Input: part model. Units: mm. Frame: model coordinates. Face numbers are marked on the shaded views. A direction names the side the tool comes from. Give positions to 0.01 mm unless a question says otherwise; leave off trailing zeros. Write each loop counter-clockwise with the first axis right and the second up, starting at its lowest first coordinate (ties: lowest second). Pieces come first, ordered by that corner, then holes.
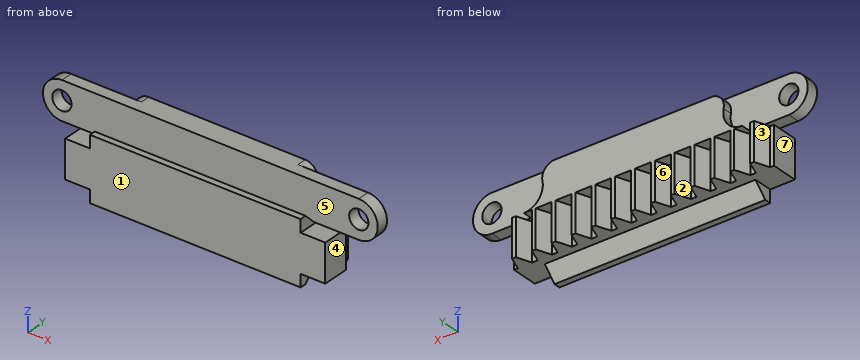
```python
from build123d import *

# Parameters (mm, degrees)
BOSS_EXTRUDE1_DEPTH              = 6
SKETCH4_W                        = 33.355842528
SKETCH4_H                        = 6
BOSS_EXTRUDE3_DEPTH              = 3
BOSS_EXTRUDE4_DEPTH              = 33.355842528
SKETCH17_W                       = 28.5
SKETCH17_H                       = 1.9
BOSS_EXTRUDE11_DEPTH             = 6
SKETCH18_R                       = 1.525
BOSS_EXTRUDE12_DEPTH             = 1.9
SKETCH20_W                       = 34.55751915
SKETCH20_H                       = 1.75
BOSS_EXTRUDE13_DEPTH             = 6
SKETCH21_R                       = 3
CUT_EXTRUDE3_DEPTH               = 1.75
FILLET2_START                    = -9.24613882
FILLET2_DEPTH                    = 1.75
BOSS_EXTRUDE14_REACH             = 49.223
SKETCH22_W                       = 6
SKETCH22_H                       = 3
BOSS_EXTRUDE14_DIRECTION_2_REACH = 49.223
SPLIT1_START                     = -66.92498259
SPLIT1_DEPTH                     = 33.355842528
SPLIT1_START_2                   = -11.14613882
SPLIT1_2_DEPTH                   = 3.65
SPLIT1_3_OUTLINE_R               = 1.525
SPLIT1_3_DEPTH                   = 1.9
SPLIT1_START_3                   = 6.755649514
SPLIT1_4_DEPTH                   = 6
SKETCH26_W                       = 6
SKETCH26_H                       = 2.5
CUT_EXTRUDE4_DEPTH               = 51.815209001
SKETCH27_W                       = 6
SKETCH27_H                       = 0.25
CUT_EXTRUDE5_DEPTH               = 80.093428855


with BuildPart() as part:
    # Sketch1 → Boss-Extrude1 (new body)
    with BuildSketch(Plane(origin=(0, 0, 0.755649514), x_dir=(-1, 0, 0), z_dir=(0, 0, -1))):
        Polygon((31.089725273, -5.24613882), (30.270792245, -7.49613882), (29.667061326, -7.49613882), (29.667061326, -11.24613882), (70.667061326, -11.24613882), (70.827061326, -11.24613882), (70.827061326, -7.49613882), (70.667061326, -7.49613882), (70.222625956, -7.49613882), (69.403692929, -5.24613882), (68.788837073, -5.24613882), (67.969904045, -7.49613882), (67.081033306, -7.49613882), (66.262100279, -5.24613882), (65.647244423, -5.24613882), (64.828311395, -7.49613882), (63.939440656, -7.49613882), (63.120507629, -5.24613882), (62.505651773, -5.24613882), (61.686718745, -7.49613882), (60.797848006, -7.49613882), (59.978914979, -5.24613882), (59.364059123, -5.24613882), (58.545126095, -7.49613882), (57.656255356, -7.49613882), (56.837322329, -5.24613882), (56.222466473, -5.24613882), (55.403533445, -7.49613882), (54.514662706, -7.49613882), (53.695729679, -5.24613882), (53.080873823, -5.24613882), (52.261940795, -7.49613882), (51.373070056, -7.49613882), (50.554137029, -5.24613882), (49.939281173, -5.24613882), (49.120348145, -7.49613882), (48.231477406, -7.49613882), (47.412544379, -5.24613882), (46.797688523, -5.24613882), (45.978755495, -7.49613882), (45.089884756, -7.49613882), (44.270951729, -5.24613882), (43.656095873, -5.24613882), (42.837162845, -7.49613882), (41.948292106, -7.49613882), (41.129359079, -5.24613882), (40.514503223, -5.24613882), (39.695570195, -7.49613882), (38.806699456, -7.49613882), (37.987766429, -5.24613882), (37.372910573, -5.24613882), (36.553977545, -7.49613882), (35.665106806, -7.49613882), (34.846173779, -5.24613882), (34.231317923, -5.24613882), (33.412384895, -7.49613882), (32.523514156, -7.49613882), (31.704581129, -5.24613882), align=None)
    extrude(amount=-BOSS_EXTRUDE1_DEPTH)

    # Sketch4 → Boss-Extrude3 (add)
    with BuildSketch(Plane.XZ.offset(11.24613882)):
        with Locations((-50.247061326, 3.755649514)):
            Rectangle(SKETCH4_W, SKETCH4_H)
    extrude(amount=BOSS_EXTRUDE3_DEPTH)

    # Sketch5 → Boss-Extrude4 (add)
    with BuildSketch(Plane.ZY.offset(66.92498259)):
        Polygon((0.755649514, -11.24613882), (-1.244350486, -13.24613882), (-1.244350486, -14.24613882), (0.755649514, -14.24613882), align=None)
        Polygon((8.755649514, -13.24613882), (8.755649514, -14.24613882), (6.755649514, -14.24613882), (6.755649514, -11.24613882), align=None)
    extrude(amount=-BOSS_EXTRUDE4_DEPTH)

    # Sketch17 → Boss-Extrude11 (add)
    with BuildSketch(Plane.XY.offset(6.755649514)):
        with Locations((-50.247061326, -10.19613882)):
            Rectangle(SKETCH17_W, SKETCH17_H)
    extrude(amount=BOSS_EXTRUDE11_DEPTH)

    # Sketch18 → Boss-Extrude12 (add)
    with BuildSketch(Plane(origin=(0, -9.24613882, 0), x_dir=(1, 0, 0), z_dir=(0, 1, 0))):
        with BuildLine():
            Line((-73.747061326, -6.755649514), (-26.747061326, -6.755649514))
            ThreePointArc((-26.747061326, -6.755649514), (-23.747061326, -9.755649514), (-26.747061326, -12.755649514))
            Line((-26.747061326, -12.755649514), (-73.747061326, -12.755649514))
            ThreePointArc((-73.747061326, -12.755649514), (-76.747061326, -9.755649514), (-73.747061326, -6.755649514))
        make_face()
        with Locations(Location((-73.747061326, -9.755649514, 0), (0, 0, 270))):
            Circle(SKETCH18_R, mode=Mode.SUBTRACT)
        with Locations(Location((-26.747061326, -9.755649514, 0), (0, 0, 270))):
            Circle(SKETCH18_R, mode=Mode.SUBTRACT)
    extrude(amount=-BOSS_EXTRUDE12_DEPTH)

    # Sketch20 → Boss-Extrude13 (add)
    with BuildSketch(Plane.XY.offset(6.755649514)):
        with Locations((-50.246709101, -8.37113882)):
            Rectangle(SKETCH20_W, SKETCH20_H)
    extrude(amount=BOSS_EXTRUDE13_DEPTH)

    # Sketch21 → Cut-Extrude3 (cut)
    with BuildSketch(Plane(origin=(0, -7.49613882, 0), x_dir=(1, 0, 0), z_dir=(0, 1, 0))):
        with Locations((-67.525468676, -9.755649514)):
            Circle(SKETCH21_R)
        with Locations((-32.967949526, -9.755649514)):
            Circle(SKETCH21_R)
    extrude(amount=-CUT_EXTRUDE3_DEPTH, mode=Mode.SUBTRACT)

    # Fillet2: read off the stored shape, not the designer's step
    # Fillet2 outline → Fillet2 (cut)
    with BuildSketch(Plane(origin=(0, 0, 0), x_dir=(1, 0, 0), z_dir=(0, 1, 0)).offset(FILLET2_START)):
        with BuildLine():
            ThreePointArc((-35.907337217, -10.355649514), (-36.317735672, -12.020560578), (-37.866929011, -12.755649514))
            Line((-37.866929011, -12.755649514), (-32.967949526, -12.755649514))
            ThreePointArc((-32.967949526, -12.755649514), (-34.865316122, -12.079439522), (-35.907337217, -10.355649514))
        make_face()
        with BuildLine():
            ThreePointArc((-62.62648919, -12.755649514), (-64.175682529, -12.020560579), (-64.586080984, -10.355649514))
            ThreePointArc((-64.586080984, -10.355649514), (-65.62810208, -12.079439522), (-67.525468676, -12.755649514))
            Line((-67.525468676, -12.755649514), (-62.62648919, -12.755649514))
        make_face()
    extrude(amount=FILLET2_DEPTH, mode=Mode.SUBTRACT)

    # Boss-Extrude14: up to this face of the body (flat: up to its plane)
    boss_extrude14_end = Plane(part.part.faces().sort_by_distance((-70.827061326, -9.37113882, 3.755649514))[0])
    # Sketch22 → Boss-Extrude14 (add, up to the picked face)
    with BuildSketch(Plane.ZY.offset(66.92498259), mode=Mode.PRIVATE) as boss_extrude14_sk1:
        with Locations((3.755649514, -12.74613882)):
            Rectangle(SKETCH22_W, SKETCH22_H)
    boss_extrude14_tool1 = split(extrude(boss_extrude14_sk1.sketch, amount=BOSS_EXTRUDE14_REACH, mode=Mode.PRIVATE), bisect_by=boss_extrude14_end, keep=Keep.BOTH, mode=Mode.PRIVATE)
    add(boss_extrude14_tool1.solids().sort_by(Axis((-66.924983, -12.746139, 3.75565), (-1, 0, 0)))[0])

    # Boss-Extrude14 direction 2: up to this face of the body (flat: up to its plane)
    boss_extrude14_direction_2_end = Plane(part.part.faces().sort_by_distance((-29.667061326, -9.37113882, 3.755649514))[0])
    # Sketch22 → Boss-Extrude14 direction 2 (add, up to the picked face)
    with BuildSketch(Plane.ZY.offset(66.92498259), mode=Mode.PRIVATE) as boss_extrude14_direction_2_sk1:
        with Locations((3.755649514, -12.74613882)):
            Rectangle(SKETCH22_W, SKETCH22_H)
    boss_extrude14_direction_2_tool1 = split(extrude(boss_extrude14_direction_2_sk1.sketch, amount=-BOSS_EXTRUDE14_DIRECTION_2_REACH, mode=Mode.PRIVATE), bisect_by=boss_extrude14_direction_2_end, keep=Keep.BOTH, mode=Mode.PRIVATE)
    add(boss_extrude14_direction_2_tool1.solids().sort_by(Axis((-66.924983, -12.746139, 3.75565), (1, 0, 0)))[0])

    # Split1 4 outline → Split1 4 (cut)
    with BuildSketch(Plane.XY.offset(SPLIT1_START_3)):
        Polygon((-66.92498259, -14.24613882), (-33.569140062, -14.24613882), (-33.569140062, -11.14613882), (-22, -11.14613882), (-22, -7.49613882), (-78, -7.49613882), (-78, -11.14613882), (-66.92498259, -11.14613882), align=None)
    extrude(amount=SPLIT1_4_DEPTH, mode=Mode.SUBTRACT)

    # Sketch26 → Cut-Extrude4 (cut, through all)
    with BuildSketch(Plane(origin=(-29.667061326, 0, 0), x_dir=(0, 0, -1), z_dir=(1, 0, 0))):
        with Locations((-3.755649514, -9.24613882)):
            Rectangle(SKETCH26_W, SKETCH26_H)
    extrude(amount=-CUT_EXTRUDE4_DEPTH, mode=Mode.SUBTRACT)


with BuildPart() as body_2:
    # Split1: read off the stored shape, not the designer's step
    # Split1 outline → Split1 (new body)
    with BuildSketch(Plane.YZ.offset(SPLIT1_START)):
        Polygon((-14.24613882, 8.755649514), (-14.24613882, 6.755649514), (-11.24613882, 6.755649514), (-13.24613882, 8.755649514), align=None)
    extrude(amount=SPLIT1_DEPTH)


with BuildPart() as body_3:
    # Split1 2 outline → Split1 2 (new body)
    with BuildSketch(Plane(origin=(0, 0, 0), x_dir=(1, 0, 0), z_dir=(0, 1, 0)).offset(SPLIT1_START_2)):
        with BuildLine():
            Line((-32.967949526, -6.755649514), (-67.525468676, -6.755649514))
            ThreePointArc((-67.525468676, -6.755649514), (-65.201678668, -7.858282918), (-64.586080984, -10.355649514))
            ThreePointArc((-64.586080984, -10.355649514), (-64.175682529, -12.020560579), (-62.62648919, -12.755649514))
            Line((-62.62648919, -12.755649514), (-37.866929011, -12.755649514))
            ThreePointArc((-37.866929011, -12.755649514), (-36.317735672, -12.020560578), (-35.907337217, -10.355649514))
            ThreePointArc((-35.907337217, -10.355649514), (-35.291739533, -7.858282918), (-32.967949526, -6.755649514))
        make_face()
    extrude(amount=SPLIT1_2_DEPTH)

    # Split1 3 outline → Split1 3 (add)
    # profile 1 of 2: a face of its own
    with BuildSketch(Plane(origin=(0, 0, 0), x_dir=(1, 0, 0), z_dir=(0, 1, 0)).offset(SPLIT1_START_2)):
        with BuildLine():
            Line((-67.525468676, -6.755649514), (-73.747061326, -6.755649514))
            ThreePointArc((-73.747061326, -6.755649514), (-76.747061326, -9.755649514), (-73.747061326, -12.755649514))
            Line((-73.747061326, -12.755649514), (-62.62648919, -12.755649514))
            ThreePointArc((-62.62648919, -12.755649514), (-64.175682529, -12.020560579), (-64.586080984, -10.355649514))
            ThreePointArc((-64.586080984, -10.355649514), (-65.201678668, -7.858282918), (-67.525468676, -6.755649514))
        make_face()
        with Locations((-73.747061326, -9.755649514)):
            Circle(SPLIT1_3_OUTLINE_R, mode=Mode.SUBTRACT)
    # profile 2 of 2: a face of its own
    with BuildSketch(Plane(origin=(0, 0, 0), x_dir=(1, 0, 0), z_dir=(0, 1, 0)).offset(SPLIT1_START_2)):
        with BuildLine():
            Line((-26.747061326, -6.755649514), (-32.967949526, -6.755649514))
            ThreePointArc((-32.967949526, -6.755649514), (-35.291739533, -7.858282918), (-35.907337217, -10.355649514))
            ThreePointArc((-35.907337217, -10.355649514), (-36.317735672, -12.020560578), (-37.866929011, -12.755649514))
            Line((-37.866929011, -12.755649514), (-26.747061326, -12.755649514))
            ThreePointArc((-26.747061326, -12.755649514), (-23.747061326, -9.755649514), (-26.747061326, -6.755649514))
        make_face()
        with Locations((-26.747061326, -9.755649514)):
            Circle(SPLIT1_3_OUTLINE_R, mode=Mode.SUBTRACT)
    extrude(amount=SPLIT1_3_DEPTH)


with BuildPart() as cut_extrude4_piece_1:
    # of the separate pieces the step leaves, piece 1, a body of its own (cut_extrude4_pieces)
    add(part.part.solids().sort_by_distance((-29.667061326, -10.49613882, 0.755649514))[0])


with BuildPart() as cut_extrude4_piece_2:
    # of the separate pieces the step leaves, piece 2, a body of its own (cut_extrude4_pieces)
    add(part.part.solids().sort_by_distance((-31.089725273, -5.24613882, 0.755649514))[0])


with BuildPart() as cut_extrude4_piece_2_1:
    # Body-Move/Copy1: read off the stored shape, not the designer's step
    # Body-Move/Copy1: moved
    add(cut_extrude4_piece_2.part.moved(Location((0, -2.5, 0))))


with BuildPart() as cut_extrude4_piece_1_1:
    add(cut_extrude4_piece_1.part)

    # Combine1: union Cut-Extrude4 piece 2, body 3, body 2
    add(cut_extrude4_piece_2_1.part)
    add(body_3.part)
    add(body_2.part)

    # Sketch27 → Cut-Extrude5 (cut, through all)
    with BuildSketch(Plane(origin=(0, 0, 0), x_dir=(0, 0, -1), z_dir=(1, 0, 0))):
        with Locations((-9.755649514, -7.62113882)):
            Rectangle(SKETCH27_W, SKETCH27_H)
    extrude(amount=-CUT_EXTRUDE5_DEPTH, mode=Mode.SUBTRACT)


solid = cut_extrude4_piece_1_1.part
```
Q1. Mould query, pull axis X, two halves, no side actions, for the marked faces 1, 2 and 3. Classes: +X half, -X half, draft (parallel to the pull), parting line (faces both ways), or undercut.
Q2. Section B-B, the plane y = -8.25. Give the number of separate pieces and of enclosed holes in the cut face, then the cut area to 3 significant figures.
Q3. Access query for the marked faces 4, 5, 6 and 7. Directions: +Z, -Z, +X, -X, +Y, -Y. A direction counts if a zero-diameter tool reaches every point of the face in a straight line with its end or side. Return the directions, or none.
Q4. Section A-A, the plane y = -12. Return the cut outline in (x, z), then the cut area to 3 significant figures.
Q5. Section C-C, the plane z = -0.5. Return the cut outline in (x, y), then the cut area to 3 significant figures.
Q6. Material intervals for line 1 along X through (y, z) = (-10.25, 11); line 2 along X through (y, z) = (-10, 10.75); line 3 along Z through (x, y) = (-64.5, -11), sorted ascending.
Q7. Pin query (flat end, axial travel): pin 1 (2 mm diameter, centred on y = -9.5, z = 1.5, fed in from +X); pin 2 (1.5 mm diameter, centred on x = -40.5, y = -10, fed in from -Z); pin 3 (3.5 mm diameter, centred on y = -11.5, z = 5, fed in from -X). Return the tip coordinate at first contact, or that it passes through.
Solutions:
1. face 1: draft
1. face 2: undercut
1. face 3: -X half
2. separate pieces: 3
2. enclosed holes: 0
2. area: 251 mm2
3. face 4: -Z, +X, +Y, -Y
3. face 5: +Z, +X, -X
3. face 6: -Z, +Y
3. face 7: -Z, -X, +Y, -Y
4. outline: (-70.83, 0.76) - (-66.92, 0.76) - (-66.92, 0) - (-33.57, 0) - (-33.57, 0.76) - (-29.67, 0.76) - (-29.67, 6.76) - (-33.57, 6.76) - (-33.57, 7.51) - (-66.92, 7.51) - (-66.92, 6.76) - (-70.83, 6.76) - close
4. area: 297 mm2
5. outline: (-66.92, -14.25) - (-33.57, -14.25) - (-33.57, -12.5) - (-66.92, -12.5) - close
5. area: 58.2 mm2
6. line 1: x = -76.48 to -74.63, -72.87 to -27.63, -25.87 to -24.02
6. line 2: x = -76.58 to -74.9, -72.59 to -27.9, -25.59 to -23.92
6. line 3: z = 0.76 to 12.76
7. pin 1: stops at x = -29.67
7. pin 2: stops at z = 0.76
7. pin 3: stops at x = -70.83
